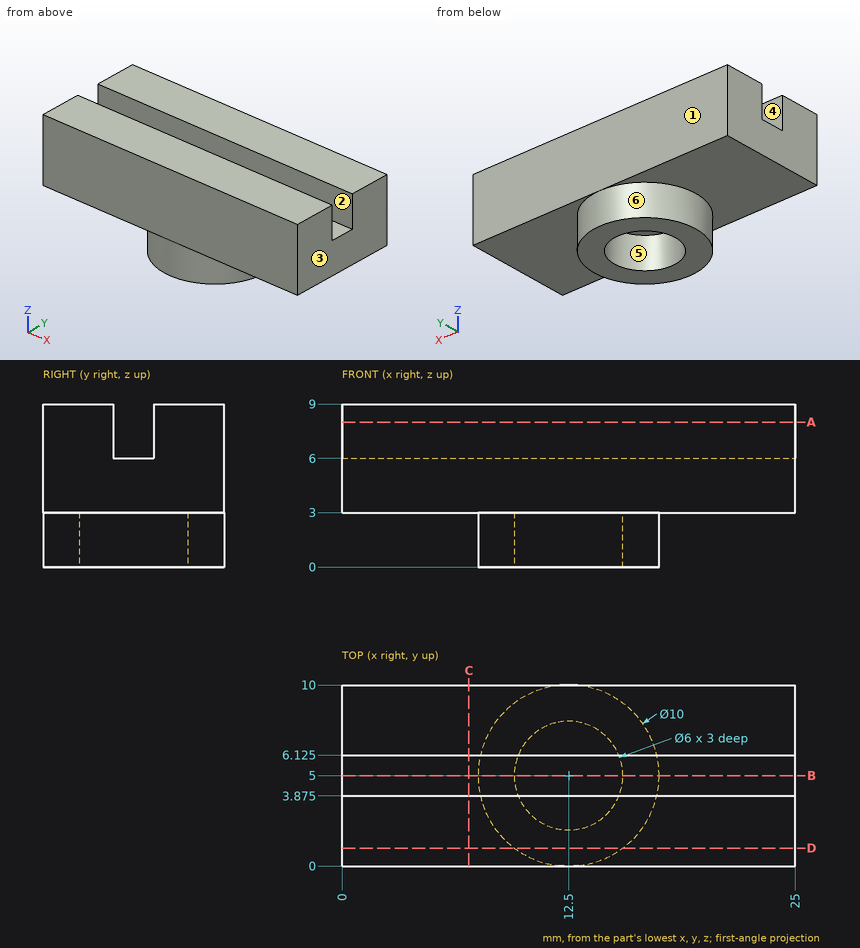
The figure shows three views and two pictorial views of one solid part (mm, origin at its lowest corner). Answer the questions. A direction names the side the tool comes from. Give positions to 0.01 mm unless a question says otherwise; leave off trailing zeros. Write each loop counter-clockwise with the first axis right and the second up, starting at its lowest first coordinate (ties: lowest second). Pieces come first, ordered by that corner, then holes. Notation, with made-up numbers: (1.5, 65.25) - (35.5, 65.25) arc R15 cw to (35.5, 94.25) - close; hole circle Ø6 at (7, -40). An arc over 180 degrees is marked (long way). Use one line per item in the form item = value. Start each with the question number.
1) Find section D-D on y = 1. Determine the outline of the cut face in (x, z).
2) Flat-ended cylindrical pins translate along their axes: pin 1 Ø0.7 at (x, y) = (11.5, 5.5) entering from +Z; pin 2 Ø2 at (y, z) = (6, 1.5) entering from +X; pin 3 Ø3 at (x, y) = (13, 6) entering from -Z. Find the tip coordinate at first contact, or state that the pin passes through.
3) Find section A-A on z = 8. Determine the outline of the cut face in (x, y) (3 decimals), plus the area to 3 significant figures.
4) Consider line 1 along Y through (x, z) = (22.5, 6.25) (3 decimals); line 2 along Y through (x, z) = (12.5, 0.9); line 3 along Z through (x, y) = (6.5, 8). Determine where each line is inside the solid, lowest interval first. Write a range as from..to.
5) A tool of negligible diameter and unlimited length cuts with its end or side. For the marked faces 1 and 2, from which of +Z, -Z, +X, -X, +Y, -Y can it reach the whole face along a straight path? Write none if from no direction.
6) Find section C-C on x = 7. Determine the outline of the cut face in (y, z) (3 decimals), plus the area to 4 significant figures.
7) Find section B-B on y = 5. Determine the outline of the cut face in (x, z), plus the area to 3 significant figures.
8) The mould has two halves that part along X. Classify the marked faces 3, 4, 5 and 6: pulls with the +X half, pulls with the -X half, needs draft (parallel to the pull), parting line crosses it, or undercut.
Geometry results:
q1.outline = (0, 3) - (9.5, 3) - (9.5, 0) - (15.5, 0) - (15.5, 3) - (25, 3) - (25, 9) - (0, 9) - close
q2.pin_1 = 6
q2.pin_2 = 17.5
q2.pin_3 = 3
q3.outline = (0, 0) - (25, 0) - (25, 3.875) - (0, 3.875) - close; (0, 6.125) - (25, 6.125) - (25, 10) - (0, 10) - close
q3.area = 194 mm2
q4.line_1 = 0..3.875, 6.125..10
q4.line_2 = 0..2, 8..10
q4.line_3 = 3..9
q5.face_1 = +Z, -Z, +X, -X, +Y
q5.face_2 = +Z, +X, -X
q6.outline = (0, 3) - (10, 3) - (10, 9) - (6.125, 9) - (6.125, 6) - (3.875, 6) - (3.875, 9) - (0, 9) - close
q6.area = 53.25 mm2
q7.outline = (0, 3) - (7.5, 3) - (7.5, 0) - (9.5, 0) - (9.5, 3) - (15.5, 3) - (15.5, 0) - (17.5, 0) - (17.5, 3) - (25, 3) - (25, 6) - (0, 6) - close
q7.area = 87.0 mm2
q8.face_3 = pulls with the +X half
q8.face_4 = needs draft
q8.face_5 = undercut
q8.face_6 = parting line crosses it
